```python
from build123d import *

# Parameters (mm, degrees)
SKETCH1_R           = 1.7
SKETCH1_RX          = 3.021964858
SKETCH1_RY          = 2.2
BOSS_EXTRUDE1_DEPTH = 2


with BuildPart() as part:
    # Sketch1 → Boss-Extrude1 (new body)
    with BuildSketch(Plane(origin=(0, 0, 0), x_dir=(0, 0, -1), z_dir=(1, 0, 0))):
        with BuildLine():
            Line((-4.7, -15.443929717), (-4.7, 0))
            ThreePointArc((-4.7, 0), (0, 4.7), (4.7, 0))
            Line((4.7, 0), (4.7, -15.443929717))
            ThreePointArc((4.7, -15.443929717), (0, -20.143929717), (-4.7, -15.443929717))
        make_face()
        Circle(SKETCH1_R, mode=Mode.SUBTRACT)
        with Locations((0, -15.443929717)):
            Circle(SKETCH1_R, mode=Mode.SUBTRACT)
        with Locations(Location((0, -7.721964858), (0, 0, -90))):
            Ellipse(SKETCH1_RX, SKETCH1_RY, mode=Mode.SUBTRACT)
    extrude(amount=BOSS_EXTRUDE1_DEPTH)


solid = part.part
```
Read the model definition and answer for the solid it produces. Units are mm, in the model's axes. Round coordinates to 2 decimals unless told otherwise and drop trailing zeros. Write each loop counter-clockwise with the first axis right and the second up, starting at its lowest first coordinate (ties: lowest second). Pieces come first, ordered by that corner, then holes. Notation, with made-up numbers: (59.5, 69) - (103.5, 69) arc R28 ccw to (103.5, 87) - close; hole circle Ø5 at (47.5, 65). An arc over 180 degrees is marked (long way). One line per item, written item: value.
Q1. Find section C-C (z = 3.25). Determine the outline of the cut face in (x, y), and give its area (3 significant figures).
The answers:
outline: (0, -18.84) - (2, -18.84) - (2, 3.4) - (0, 3.4) - close
area: 44.5 mm2
Q2. For a pull along Z with two mould halves and no side action, classify faces 1 (the cylindrical face through (0.99, -1.66, 0.37)), 2 (the flat face through (1, -8, 4.7)), 3 (the flat face through (0, -4.8, 1)) as pulls with the +Z half, pulls with the -Z half, needs draft (parallel to the pull), parting line crosses it, or undercut.
The answers:
face 1: undercut
face 2: pulls with the +Z half
face 3: needs draft
Q3. Find section A-A (z = 0). Count the separate pieces of the cut face and the enclosed holes in it, and give its area (3 significant figures).
The answers:
separate pieces: 4
enclosed holes: 0
area: 24.0 mm2
Q4. This flat-tipped pin is pushed along its axis until it touches: P1, Ø2, axis at y = -15.44, z = 0, coming from the -X side. Where does it stop, or does it pass through?
The answers:
P1: passes through
Q5. Find section D-D (z = -2.5). Determine the outline of the cut face in (x, y).
The answers:
outline: (0, -19.42) - (2, -19.42) - (2, 3.98) - (0, 3.98) - close
Q6. Straight lines are drawn through the part: line 1 (Y direction, x = 1, z = 0); line 2 (Z direction, x = 0.65, y = -7.75); line 3 (Y direction, x = 0.9, z = 1.5). For each, find the intervals that lie inside material, in ascending order. Write a range as from..to.
The answers:
line 1: y = -20.14..-17.14, -13.74..-10.74, -4.7..-1.7, 1.7..4.7
line 2: z = -4.7..-2.2, 2.2..4.7
line 3: y = -19.9..-16.24, -14.64..-9.93, -5.51..-0.8, 0.8..4.45
